from build123d import *

# Parameters (mm, degrees)
PAD_DEPTH       = 25.4
SKETCH001_R     = 2.413
POCKET_DEPTH    = 10.16
SKETCH002_R     = 2.413
POCKET001_DEPTH = 10.16
SKETCH003_W     = 3.302
SKETCH003_H     = 12.7
POCKET002_DEPTH = 20.32
SKETCH004_W     = 1.963636
SKETCH004_H     = 12.7
POCKET003_DEPTH = 20.32


with BuildPart() as part:
    # Sketch → Pad (new body)
    with BuildSketch(Plane.XY):
        with BuildLine():
            Line((25.4, 0), (0, 0))
            Line((0, 3.048), (0, 0))
            Line((0, 3.048), (2.032, 3.048))
            Line((2.032, 3.048), (2.032, 28.448))
            Line((2.032, 28.448), (-3.048, 28.448))
            Line((-3.048, 28.448), (-6.35, 3.048))
            ThreePointArc((-6.35, 3.048), (-5.961619, -3.751253), (0, -7.043636))
            Line((0, -7.043636), (25.4, -5.08))
            Line((25.4, 0), (25.4, -5.08))
        make_face()
    extrude(amount=PAD_DEPTH)

    # Sketch001 (on Face4 of Pad) → Pocket (cut)
    with BuildSketch(Plane.YZ.offset(2.032)):
        with Locations((15.748, 12.7)):
            Circle(SKETCH001_R)
    extrude(amount=-POCKET_DEPTH, mode=Mode.SUBTRACT)

    # Sketch002 (on Face1 of Pocket) → Pocket001 (cut)
    with BuildSketch(Plane(origin=(0, 0, 0), x_dir=(-1, 0, 0), z_dir=(0, 1, 0))):
        with Locations((-12.7, 12.7)):
            Circle(SKETCH002_R)
    extrude(amount=-POCKET001_DEPTH, mode=Mode.SUBTRACT)

    # Sketch003 (on Face10 of Pocket001) → Pocket002 (cut)
    with BuildSketch(Plane(origin=(0, 28.448, 0), x_dir=(-1, 0, 0), z_dir=(0, 1, 0))):
        with Locations((4.699, 12.7)):
            Rectangle(SKETCH003_W, SKETCH003_H)
    extrude(amount=-POCKET002_DEPTH, mode=Mode.SUBTRACT)

    # Sketch004 (on Face2 of Pocket002) → Pocket003 (cut)
    with BuildSketch(Plane.YZ.offset(25.4)):
        with Locations((-6.061818, 12.7)):
            Rectangle(SKETCH004_W, SKETCH004_H)
    extrude(amount=-POCKET003_DEPTH, mode=Mode.SUBTRACT)


solid = part.part
Build history of the part. All positions in model axes, mm. A direction names the side the tool comes from. Coordinates: 2 decimals unless noted, no trailing zeros. Order: outer loops, then holes, each group sorted by start corner. A loop starts at its lowest first (then second) coordinate and runs counter-clockwise, first axis right, second up. Notation, with made-up numbers: (28.5, -37.5) - (60.5, -37.5) arc R38 cw to (60.5, 1.5) - close; hole circle Ø10 at (88, 7). An arc over 180 degrees is marked (long way). Write item = value, one per line. Start each with the question number.
1) Flat gauge pins, fed straight in: pin 1 Ø1.5 at (x, z) = (21, 22) entering from -Y; pin 2 Ø7.5 at (y, z) = (15.748, 12.7) entering from -X; pin 3 Ø1 at (x, z) = (5.5, 16.5) entering from +Y; pin 4 Ø10 at (x, y) = (9.5, 22) entering from +Z. Where does each tip first touch, or does it go through?
2) Saw through at C-C on y = 14. Write the cut outline in (x, z).
3) Saw through at D-D on z = 4.5. Write the cut outline in (x, y).
4) 3-axis set-ups, long thin cutter, end or side, ignore diameter. For faces 1 (the face through (2.032, 18.4, 12.5)), 2 (the face through (11, -6, 6.35)), 3 (the face through (-4, 14, 19.05)): which of +Z, -Z, +X, -X, +Y, -Y reach the whole face in a straight line?
5) Two-plate mould, pull along X, no slides. Class faces 4 (the face through (11.587, -2.504, 10.559)), 5 (the face through (-6.01, -3.67, 12.52)), 6 (the face through (-4, 8.128, 13)): pulls with the +X half, pulls with the -X half, needs draft (parallel to the pull), parting line crosses it, or undercut.
6) Saw through at A-A on z = 12.7. Write the cut outline in (x, y) (3 decimals), then the cut area to 3 significant figures.
7) Wall check: line 1 along Z through (x, y) = (12.7, -2.7); line 2 along Y through (x, z) = (1, 14.25); line 3 along X through (y, z) = (13, 18). Give the ranges that are in metal, low to high. Write a range as from..to.
8) Saw through at B-B on x = 12.7. Write the cut outline in (y, z), then the cut area to 3 significant figures.
From the geometry:
q1.pin_1 = -5.48
q1.pin_2 = -3.05
q1.pin_3 = 0
q1.pin_4 = through
q2.outline = (-4.93, 0) - (2.03, 0) - (2.03, 11.04) - (-3.05, 11.04) - (-3.05, 6.35) - (-4.93, 6.35) - close; (-4.93, 19.05) - (-3.05, 19.05) - (-3.05, 14.36) - (2.03, 14.36) - (2.03, 25.4) - (-4.93, 25.4) - close
q3.outline = (-6.35, 3.05) arc R7.04 ccw to (0, -7.04) - (25.4, -5.08) - (25.4, 0) - (0, 0) - (0, 3.05) - (2.03, 3.05) - (2.03, 28.45) - (-3.05, 28.45) - close
q4.face_1 = +Z, -Z, +X, +Y
q4.face_2 = +X, -Y
q4.face_3 = -X, +Y
q5.face_4 = undercut
q5.face_5 = pulls with the -X half
q5.face_6 = needs draft
q6.outline = (-6.35, 3.048) arc R7.044 ccw to (0, -7.044) - (5.08, -6.651) - (5.08, -5.08) - (10.287, -5.08) - (10.287, 0) - (0, 0) - (0, 3.048) - (2.032, 3.048) - (2.032, 13.335) - (-3.048, 13.335) - (-3.048, 8.128) - (-5.69, 8.128) - close; (-3.048, 18.161) - (2.032, 18.161) - (2.032, 28.448) - (-3.048, 28.448) - close; (15.113, -5.08) - (25.4, -5.08) - (25.4, 0) - (15.113, 0) - close
q6.area = 293 mm^2
q7.line_1 = 0..10.29, 15.11..25.4
q7.line_2 = -6.97..0, 3.05..13.9, 17.6..28.45
q7.line_3 = -3.05..2.03
q8.outline = (-6.06, 0) - (0, 0) - (0, 10.29) - (-5.08, 10.29) - (-5.08, 6.35) - (-6.06, 6.35) - close; (-6.06, 19.05) - (-5.08, 19.05) - (-5.08, 15.11) - (0, 15.11) - (0, 25.4) - (-6.06, 25.4) - close
q8.area = 117 mm^2
